Geometry check sheet. Reference: the model listing, model coordinates, mm. Round coordinates to 2 decimals unless told otherwise and drop trailing zeros. Write each loop counter-clockwise with the first axis right and the second up, starting at its lowest first coordinate (ties: lowest second). Pieces come first, ordered by that corner, then holes. Notation, with made-up numbers: M 19.25,-34.75 L 71.25,-34.75 A15 ccw 71.25,-18.75 Z; hole C 39,40.5 d4. An arc over 180 degrees is marked long. Answer in a Markdown table with one row per item. Add a question column.
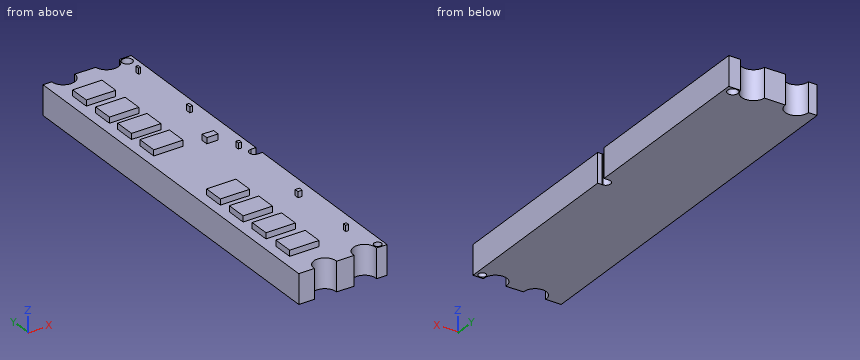
from build123d import *

# Parameters (mm, degrees)
F1_DEPTH = 1
F2_R     = 0.174096
F2_R_2   = 0.127508
F3_DEPTH = 1.001
F4_W     = 1
F4_H     = 0.7
F4_W_2   = 0.384185
F4_H_2   = 0.232839
F5_DEPTH = 0.2
F7_DEPTH = 1.001
F8_W     = 0.069853
F8_H     = 0.121337
F8_W_2   = 0.093136
F8_H_2   = 0.169292
F8_W_3   = 0.105232
F8_H_3   = 0.113234
F8_W_4   = 0.097446
F8_H_4   = 0.104777
F8_W_5   = 0.144014
F8_H_5   = 0.139706
F9_DEPTH = 0.2


with BuildPart() as f1:
    # F0 (on Top) → F1 (new body)
    with BuildSketch(Plane.XY):
        with BuildLine():
            Line((-24.902489, -49.29686), (-25.199003, -49.29686))
            Line((-25.199003, -49.29686), (-25.199003, -62.29686))
            Line((-25.199003, -62.29686), (-24.669482, -62.29686))
            ThreePointArc((-24.669482, -62.29686), (-24.2913, -61.893387), (-23.913119, -62.29686))
            Line((-23.913119, -62.29686), (-23.314611, -62.29686))
            ThreePointArc((-23.314611, -62.29686), (-22.93501, -61.872911), (-22.55541, -62.29686))
            Line((-22.55541, -62.29686), (-22.199003, -62.29686))
            Line((-22.199003, -62.29686), (-22.199003, -49.29686))
            Line((-22.199003, -49.29686), (-22.603517, -49.29686))
            ThreePointArc((-22.603517, -49.29686), (-23.008304, -49.655694), (-23.41309, -49.29686))
            Line((-23.41309, -49.29686), (-24.119699, -49.29686))
            ThreePointArc((-24.119699, -49.29686), (-24.511094, -49.688254), (-24.902489, -49.29686))
        make_face()
    extrude(amount=F1_DEPTH)

    # F2 (on Top) → F3 (cut, through all)
    with BuildSketch(Plane.XY):
        with Locations((-22.469135, -49.496643)):
            Circle(F2_R)
        with Locations((-22.408167, -62.138651)):
            Circle(F2_R_2)
    extrude(amount=F3_DEPTH, mode=Mode.SUBTRACT)

    # F4 (on face) → F5 (join)
    with BuildSketch(Plane.XY.offset(1)):
        with Locations((-24.362976, -50.646318)):
            Rectangle(F4_W, F4_H)
        with Locations((-24.362976, -51.822787)):
            Rectangle(F4_W, F4_H)
        with Locations((-24.362976, -52.940436)):
            Rectangle(F4_W, F4_H)
        with Locations((-24.362976, -54.072786)):
            Rectangle(F4_W, F4_H)
        with Locations((-23.037707, -54.56131)):
            Rectangle(F4_W_2, F4_H_2)
        with Locations((-24.362976, -60.980084)):
            Rectangle(F4_W, F4_H)
        with Locations((-24.362976, -59.776055)):
            Rectangle(F4_W, F4_H)
        with Locations((-24.362976, -58.616622)):
            Rectangle(F4_W, F4_H)
        with Locations((-24.362976, -57.457188)):
            Rectangle(F4_W, F4_H)
    extrude(amount=F5_DEPTH)

    # F6 (on face) → F7 (cut, through all)
    with BuildSketch(Plane.XY.offset(1)):
        with BuildLine():
            Line((-22.353487, -55.96097), (-22.373339, -55.96097))
            ThreePointArc((-22.373339, -55.96097), (-22.363413, -55.96127), (-22.353487, -55.96097))
        make_face()
        with BuildLine():
            Line((-22.199003, -55.63259), (-22.363273, -55.63245))
            ThreePointArc((-22.363273, -55.63245), (-22.527746, -55.791824), (-22.373339, -55.96097))
            Line((-22.373339, -55.96097), (-22.353487, -55.96097))
            Line((-22.353487, -55.96097), (-22.199003, -55.96097))
            Line((-22.199003, -55.96097), (-22.199003, -55.63259))
        make_face()
    extrude(amount=-F7_DEPTH, mode=Mode.SUBTRACT)

    # F8 (on face) → F9 (join)
    with BuildSketch(Plane.XY.offset(1)):
        with Locations((-22.587573, -50.235649)):
            Rectangle(F8_W, F8_H)
        with Locations((-22.599215, -52.85579)):
            Rectangle(F8_W_2, F8_H_2)
        with Locations((-22.605263, -55.366989)):
            Rectangle(F8_W_3, F8_H_3)
        with Locations((-22.706602, -60.973562)):
            Rectangle(F8_W_4, F8_H_4)
        with Locations((-22.729886, -58.604419)):
            Rectangle(F8_W_5, F8_H_5)
    extrude(amount=F9_DEPTH)


solid = f1.part
Item 1: Scan lines: probe 1 along Z at (x, y) = (-24.9, -50); probe 2 along Y at (x, z) = (-23.35, 0.1); probe 3 along Y at (x, z) = (-24.4, 0.3). Record each from-to range of solid material in increasing order. Write a range as from..to.
Item 2: Section check D-D, the plane y = -57. Record the boundary of the cut face in (x, z), and give its area (3 significant figures).
Item 3: Section check A-A, the plane y = -60. Record the boundary of the cut face in (x, z).
Item 4: Section check C-C, the plane x = -23.65. Record the boundary of the cut face in (y, z), and give its area (3 significant figures).
Item 5: Section check B-B, the plane z = 0.25. Give the number of separate pieces and of enclosed holes in the cut face, and give its area (3 significant figures).
Result sheet:
| question | item | result |
|---|---|---|
| 1 | probe 1 | z = 0..1 |
| 1 | probe 2 | y = -62.3..-49.47 |
| 1 | probe 3 | y = -61.91..-49.67 |
| 2 | outline | M -25.2,0 L -22.2,0 L -22.2,1 L -25.2,1 Z |
| 2 | area | 3.00 mm^2 |
| 3 | outline | M -25.2,0 L -22.2,0 L -22.2,1 L -23.86,1 L -23.86,1.2 L -24.86,1.2 L -24.86,1 L -25.2,1 Z |
| 4 | outline | M -62.3,0 L -49.3,0 L -49.3,1 L -62.3,1 Z |
| 4 | area | 13.0 mm^2 |
| 5 | separate pieces | 1 |
| 5 | enclosed holes | 2 |
| 5 | area | 37.8 mm^2 |
